from build123d import *

# Parameters (mm, degrees)
F0_W     = 46.99
F0_H     = 46.99
F0_W_2   = 44.45
F0_H_2   = 44.45
F0_W_3   = 31.75
F0_H_3   = 31.75
F1_DEPTH = 25.4
F2_DEPTH = 4.7625


with BuildPart() as f1:
    # F0 (on Top) → F1 (new body)
    with BuildSketch(Plane.XY):
        with Locations((-23.495, 23.495)):
            Rectangle(F0_W, F0_H)
        with Locations((-23.495, 23.495)):
            Rectangle(F0_W_2, F0_H_2, mode=Mode.SUBTRACT)
        with Locations((-23.495, 23.495)):
            Rectangle(F0_W_2, F0_H_2)
        with Locations((-23.495, 23.495)):
            Rectangle(F0_W_3, F0_H_3, mode=Mode.SUBTRACT)
        with Locations((-23.495, 23.495)):
            Rectangle(F0_W_3, F0_H_3)
    extrude(amount=-F1_DEPTH)

    # F0 (on Top) → F2 (cut)
    with BuildSketch(Plane.XY):
        with Locations((-23.495, 23.495)):
            Rectangle(F0_W_2, F0_H_2)
        with Locations((-23.495, 23.495)):
            Rectangle(F0_W_3, F0_H_3, mode=Mode.SUBTRACT)
    extrude(amount=-F2_DEPTH, mode=Mode.SUBTRACT)


solid = f1.part
The listing builds one solid part. Answer for the finished solid, in the listing's coordinates (mm). A direction names the side the tool comes from. Coordinates: 2 decimals unless noted, no trailing zeros. Write each loop counter-clockwise with the first axis right and the second up, starting at its lowest first coordinate (ties: lowest second). Pieces come first, ordered by that corner, then holes. Notation, with made-up numbers: M -25.75,-27.5 L 22.25,-27.5 A29 cw 22.25,4.5 Z; hole C -23,-30.75 d4. An arc over 180 degrees is marked long. Use one line per item in the form item = value.
Item 1: Find section D-D, the plane y = 43. Give the vertices of the cut face in (x, z).
Model answer:
outline = M -46.99,-25.4 L 0,-25.4 L 0,0 L -1.27,0 L -1.27,-4.76 L -45.72,-4.76 L -45.72,0 L -46.99,0 Z
Item 2: Find section A-A, the plane y = 24.5. Give the vertices of the cut face in (x, z), plus the area to 3 significant figures.
Model answer:
outline = M -46.99,-25.4 L 0,-25.4 L 0,0 L -1.27,0 L -1.27,-4.76 L -7.62,-4.76 L -7.62,0 L -39.37,0 L -39.37,-4.76 L -45.72,-4.76 L -45.72,0 L -46.99,0 Z
area = 1,130 mm2
Item 3: Find section B-B, the plane x = -17.5. Give the vertices of the cut face in (y, z), plus the area to 3 significant figures.
Model answer:
outline = M 0,-25.4 L 46.99,-25.4 L 46.99,0 L 45.72,0 L 45.72,-4.76 L 39.37,-4.76 L 39.37,0 L 7.62,0 L 7.62,-4.76 L 1.27,-4.76 L 1.27,0 L 0,0 Z
area = 1,130 mm2
Item 4: For faces 4 (the face through (-24, 24, 0)), 5 (the face through (-24, 1.27, -2)), determine the directions among +Z, -Z, +X, -X, +Y, -Y from which every point of the face is accessible in a straight line to the end or side of a thin tool.
Model answer:
face_4 = +Z, +X, -X, +Y, -Y
face_5 = +Z
Item 5: Find section C-C, the plane x = -40.5. Give the vertices of the cut face in (y, z), plus the area to 3 significant figures.
Model answer:
outline = M 0,-25.4 L 46.99,-25.4 L 46.99,0 L 45.72,0 L 45.72,-4.76 L 1.27,-4.76 L 1.27,0 L 0,0 Z
area = 982 mm2
Item 6: The mould has two halves that part along X. Classify faces 1 (the face through (-24, 46.99, -13)), 2 (the face through (-24, 45.72, -2)), 3 (the face through (-46.99, 23, -13)): released by +X, released by -X, zero draft, split by the parting line, or undercut.
Model answer:
face_1 = zero draft
face_2 = undercut
face_3 = released by -X
Item 7: Find the intervals of material crossed by probe 1 along Y at (x, z) = (-20, -4.5); probe 2 along Y at (x, z) = (-3.5, -2); probe 3 along Z at (x, y) = (-8, 4.5), in increasing order.
Model answer:
probe_1 = 0 to 1.27, 7.62 to 39.37, 45.72 to 46.99
probe_2 = 0 to 1.27, 45.72 to 46.99
probe_3 = -25.4 to -4.76
